from build123d import *

# Parameters (mm, degrees)
RESSALTO_EXTRUS_O1_DEPTH                             = 6
ESBO_O2_W                                            = 11
ESBO_O2_H                                            = 30.1
RESSALTO_EXTRUS_O2_DEPTH                             = 28
ESBO_O3_W                                            = 13
ESBO_O3_H                                            = 30.1
RESSALTO_EXTRUS_O3_DEPTH                             = 30
REBAIXO_PARA_PARAFUSO_DE_M_QUINA_COM_CAB_D           = 6.6
REBAIXO_PARA_PARAFUSO_DE_M_QUINA_COM_CAB_CBORE_D     = 13
REBAIXO_PARA_PARAFUSO_DE_M_QUINA_COM_CAB_CBORE_DEPTH = 4.6
ESBO_O7_W                                            = 6
ESBO_O7_H                                            = 30
RESSALTO_EXTRUS_O4_DEPTH                             = 52


with BuildPart() as part:
    # Esboço1 → Ressalto-extrusão1 (new body)
    with BuildSketch(Plane.XY):
        Polygon((59.5, -82.5), (-70.5, -82.5), (-70.5, -52.5), (59.5, -52.5), (66.5, -52.5), (66.5, -82.5), align=None)
    extrude(amount=RESSALTO_EXTRUS_O1_DEPTH)

    # Esboço2 → Ressalto-extrusão2 (add)
    with BuildSketch(Plane(origin=(0, 0, 0), x_dir=(-1, 0, 0), z_dir=(0, 0, -1))):
        with Locations((65, -67.55)):
            Rectangle(ESBO_O2_W, ESBO_O2_H)
    extrude(amount=RESSALTO_EXTRUS_O2_DEPTH)

    # Esboço3 → Ressalto-extrusão3 (add)
    with BuildSketch(Plane.ZY.offset(70.5)):
        with Locations((-21.5, -67.55)):
            Rectangle(ESBO_O3_W, ESBO_O3_H)
    extrude(amount=RESSALTO_EXTRUS_O3_DEPTH)

    # Rebaixo para parafuso de máquina com cabeça panela de M61 (through all)
    with Locations(Plane(origin=(-85.492891977, -67.55, -28), x_dir=(-1, 0, 0), z_dir=(0, 0, -1))):
        with Locations((0, 0)):
            CounterBoreHole(REBAIXO_PARA_PARAFUSO_DE_M_QUINA_COM_CAB_D / 2, REBAIXO_PARA_PARAFUSO_DE_M_QUINA_COM_CAB_CBORE_D / 2, REBAIXO_PARA_PARAFUSO_DE_M_QUINA_COM_CAB_CBORE_DEPTH)

    # Esboço7 → Ressalto-extrusão4 (add)
    with BuildSketch(Plane(origin=(0, 0, 0), x_dir=(-1, 0, 0), z_dir=(0, 0, -1))):
        with Locations((-63.5, -67.5)):
            Rectangle(ESBO_O7_W, ESBO_O7_H)
    extrude(amount=RESSALTO_EXTRUS_O4_DEPTH)


solid = part.part
Geometry: final body of the model. Coordinates: model frame, mm. A direction names the side the tool comes from. Give positions to 0.01 mm unless a question says otherwise; leave off trailing zeros. Write each loop counter-clockwise with the first axis right and the second up, starting at its lowest first coordinate (ties: lowest second). Pieces come first, ordered by that corner, then holes. Notation, with made-up numbers: (82.25, -5.5) - (124.25, -5.5) arc R19 ccw to (124.25, 20.5) - close; hole circle Ø2 at (51.25, 10). An arc over 180 degrees is marked (long way). Return JSON: item names as keys, results as strings. Group by question number.
1) First-contact query: P1, Ø9, axis at x = -17.5, y = -61.5, coming from the -Z side; P2, Ø14.5, axis at x = -86, y = -65.5, coming from the -Z side; P3, Ø6, axis at x = -85.49, y = -67.55, coming from the -Z side. Flat tips, straight axial feed; report the tip coordinate or a pass-through.
2) Mould query, pull axis X, two halves, no side actions, for faces 1 (the flat face through (-82, -68, -15)), 2 (the flat face through (-100.5, -67, -22)), 3 (the flat face through (-59.5, -68, -14)). Classes: released by +X, released by -X, zero draft, split by the parting line, or undercut.
3) Set-up query: faces 4 (the flat face through (-79.7, -71.1, -28)), 5 (the flat face through (-88, -70, -23.4)), 6 (the flat face through (60.5, -68, -26)). Return all of +Z, -Z, +X, -X, +Y, -Y with unobstructed straight access to the full face (end or side cutting, diameter ignored); none if empty.
4) Line query: line 1 (X direction, y = -67, z = -25); line 2 (X direction, y = -58.5, z = -9); line 3 (Z direction, x = -43, y = -80.5). Output: solid intervals per line, ascending.
5) Section A-A on z = -20.5. Return the cut outline in (x, y), plus the area to 3 significant figures.
6) Section C-C on z = -12. Return the cut outline in (x, y), plus the area to 3 significant figures.
7) Section D-D on x = -86. Return the cut outline in (y, z), plus the area to 3 significant figures.
8) Section B-B on y = -67.55. Return the cut outline in (x, z).
Filled in:
{
 "1": {"P1": "stops at z = 0", "P2": "stops at z = -28", "P3": "passes through"},
 "2": {"face 1": "zero draft", "face 2": "released by -X", "face 3": "undercut"},
 "3": {"face 4": "-Z, -X, +Y, -Y", "face 5": "-Z", "face 6": "-Z, +Y, -Y"},
 "4": {"line 1": "x = -100.5 to -91.97, -79.02 to -59.5, 60.5 to 66.5", "line 2": "x = -70.5 to -59.5, 60.5 to 66.5", "line 3": "z = 0 to 6"},
 "5": {"outline": "(-100.5, -82.6) - (-59.5, -82.6) - (-59.5, -52.5) - (-100.5, -52.5) - close; (60.5, -82.5) - (66.5, -82.5) - (66.5, -52.5) - (60.5, -52.5) - close; hole circle Ø6.6 at (-85.49, -67.55)", "area": "1,380 mm^2"},
 "6": {"outline": "(-70.5, -82.6) - (-59.5, -82.6) - (-59.5, -52.5) - (-70.5, -52.5) - close; (60.5, -82.5) - (66.5, -82.5) - (66.5, -52.5) - (60.5, -52.5) - close", "area": "511 mm^2"},
 "7": {"outline": "(-82.6, -28) - (-74.03, -28) - (-74.03, -23.4) - (-70.81, -23.4) - (-70.81, -15) - (-82.6, -15) - close; (-64.29, -23.4) - (-61.07, -23.4) - (-61.07, -28) - (-52.5, -28) - (-52.5, -15) - (-64.29, -15) - close", "area": "277 mm^2"},
 "8": {"outline": "(-100.5, -28) - (-91.99, -28) - (-91.99, -23.4) - (-88.79, -23.4) - (-88.79, -15) - (-100.5, -15) - close; (-82.19, -23.4) - (-78.99, -23.4) - (-78.99, -28) - (-59.5, -28) - (-59.5, 0) - (60.5, 0) - (60.5, -52) - (66.5, -52) - (66.5, 6) - (-70.5, 6) - (-70.5, -15) - (-82.19, -15) - close"}
}
